from build123d import *

# Parameters (mm, degrees)
F1_DEPTH = 15.875
F2_W     = 53.975
F2_H     = 107.95
F3_DEPTH = 76.2
F4_R     = 19.05
F5_DEPTH = 76.2
F7_DEPTH = 76.2
F8_R     = 7.9375
F9_DEPTH = 25.4


with BuildPart() as f1:
    # F0 (on Top) → F1 (new body)
    with BuildSketch(Plane.XY):
        Polygon((0, 127), (0, 0), (0, -57.15), (53.975, -57.15), (53.975, 127), align=None)
    extrude(amount=F1_DEPTH)

    # F2 (on face) → F3 (join)
    with BuildSketch(Plane.XY.offset(15.875)):
        with Locations((26.9875, 34.925)):
            Rectangle(F2_W, F2_H)
    extrude(amount=F3_DEPTH)

    # F4 (on face) → F5 (cut)
    with BuildSketch(Plane.YZ.offset(53.975)):
        with Locations((34.925, 49.2125)):
            Circle(F4_R)
    extrude(amount=-F5_DEPTH, mode=Mode.SUBTRACT)

    # F6 (on face) → F7 (cut)
    with BuildSketch(Plane.XY.offset(15.875)):
        with BuildLine():
            ThreePointArc((26.9875, 111.476155), (21.37484, 97.925995), (34.925, 103.538655))
            ThreePointArc((34.925, 103.538655), (32.60016, 109.151315), (26.9875, 111.476155))
        make_face()
    extrude(amount=-F7_DEPTH, mode=Mode.SUBTRACT)

    # F8 (on face) → F9 (cut)
    with BuildSketch(Plane.XY.offset(15.875)):
        with Locations((26.9875, -33.688782)):
            Circle(F8_R)
    extrude(amount=-F9_DEPTH, mode=Mode.SUBTRACT)


solid = f1.part
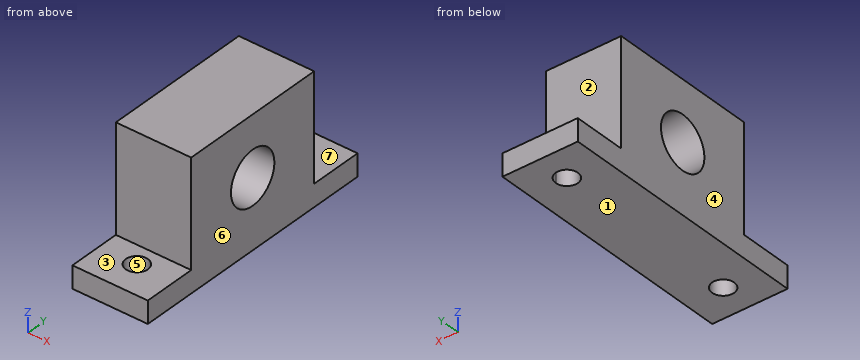
Can you work these out from the model? Positions are in its coordinate system, mm. Face numbers are marked on the shaded views. A direction names the side the tool comes from. Coordinates: 2 decimals unless noted, no trailing zeros. Loops run counter-clockwise (first coordinate to the right, second up) from the corner with the lowest first, then second, coordinate; pieces in that order, holes last. Notation, with made-up numbers: (83, 77) - (119, 77) arc R35 ccw to (119, 109) - close; hole circle Ø6 at (3.25, -7.5). An arc over 180 degrees is marked (long way). Put each result on its own line as item: value. Start each with the question number.
Item 1: If we mould it in two halves opening along X, with no side actions, what happens to the marked faces 4, 5, 6 and 7? For each: +X half, -X half, draft (parallel to the pull), parting line (faces both ways), or undercut.
Item 2: If I drill on line 1 along Z through (x, y) = (10, 36) (3 decimals); line 2 along Z through (x, y) = (17, -27) (3 decimals); line 3 along X through (y, z) = (97, 8) (3 decimals), over which ranges is the centre line in solid material (lowest first)?
Item 3: Which directions (+Z, -Z, +X, -X, +Y, -Y) give clear straight access to the entire face, cutting with the end or side of a thin tool? Please do the marked faces 1, 2 and 3.
Item 4: Suppose I cut it at D-D (z = 26). Please give me the cut outline in (x, y) (3 decimals).
Item 5: Suppose I cut it at A-A (z = 36.5). Please give me the cut outline in (x, y) (3 decimals).
Item 6: For pin 1 (18.5 mm diameter, centred on x = 26.99, y = 103.54, fed in from +Z) (3 decimals); pin 2 (1.5 mm diameter, centred on x = 24.5, z = 46.5, fed in from -Y); pin 3 (4 mm diameter, centred on y = 12, z = 53.5, fed in from -X); pin 4 (16 mm diameter, centred on x = 19, z = 59, fed in from +Y), each with a flat end and sliding along its axis, tell me the tip position at first contact or that it passes through.
Item 7: Suppose I cut it at B-B (y = 24). Please give me the cut outline in (x, z) (3 decimals).
Here are the results:
1. face 4: -X half
1. face 5: undercut
1. face 6: +X half
1. face 7: draft
2. line 1: 0 to 30.193, 68.232 to 92.075
2. line 2: 0 to 15.875
2. line 3: 0 to 22.488, 31.487 to 53.975
3. face 1: -Z, +X, -X, +Y, -Y
3. face 2: +Z, +X, -X, +Y
3. face 3: +Z, +X, -X, -Y
4. outline: (0, -19.05) - (53.975, -19.05) - (53.975, 88.9) - (0, 88.9) - close
5. outline: (0, -19.05) - (53.975, -19.05) - (53.975, 20.737) - (0, 20.737) - close; (0, 49.113) - (53.975, 49.113) - (53.975, 88.9) - (0, 88.9) - close
6. pin 1: z = 15.875
6. pin 2: y = -19.05
6. pin 3: x = 0
6. pin 4: y = 88.9
7. outline: (0, 0) - (53.975, 0) - (53.975, 33.607) - (0, 33.607) - close; (0, 64.818) - (53.975, 64.818) - (53.975, 92.075) - (0, 92.075) - close
